CAD build for the part. Positions are in the model's coordinates, mm. Face numbers are marked on the shaded views. Round coordinates to 2 decimals unless told otherwise and drop trailing zeros. Loops run counter-clockwise (first coordinate to the right, second up) from the corner with the lowest first, then second, coordinate; pieces in that order, holes last. Notation, with made-up numbers: M 37.5,60 L 65.5,60 A12 ccw 65.5,73 Z; hole C 79.25,-5 d3. An arc over 180 degrees is marked long. One line per item, written item: value. Start each with the question number.
from build123d import *

# Parameters (mm, degrees)
ESQUISSE1_W             = 120
ESQUISSE1_H             = 120
BOSS_EXTRU_2_DEPTH      = 5
ESQUISSE9_R             = 4
BOSS_EXTRU_4_DEPTH      = 37.5
CHANFREIN5_SIZE         = 15
CHANFREIN6_SIZE         = 15
CHANFREIN7_SIZE         = 15
CHANFREIN8_SIZE         = 15
D_GAGEMENT_61_D         = 2.75
D_GAGEMENT_61_DEPTH     = 15
D_GAGEMENT_61_TIP       = 0.826183351
ESQUISSE21_W            = 90
ESQUISSE21_H            = 5
BOSS_EXTRU_7_DEPTH      = 40
ESQUISSE22_W            = 90
ESQUISSE22_H            = 5
BOSS_EXTRU_8_DEPTH      = 40
CHANFREIN23_SIZE        = 20
ESQUISSE23_R            = 2
ENL_V_MAT_EXTRU_1_DEPTH = 10
SKETCH1_W               = 10
SKETCH1_H               = 55
CUT_EXTRUDE2_DEPTH      = 5
FILLET2_R               = 5
FILLET3_R               = 5
SKETCH3_W               = 10
SKETCH3_H               = 55
CUT_EXTRUDE4_DEPTH      = 5
FILLET11_R              = 5
SKETCH2_W               = 8
SKETCH2_H               = 55
CUT_EXTRUDE5_DEPTH      = 8
SKETCH4_W               = 8
SKETCH4_H               = 55
CUT_EXTRUDE6_DEPTH      = 8
FILLET12_R              = 4
FILLET13_R              = 6
FILLET14_R              = 4
FILLET15_R              = 4
SKETCH5_W               = 3
SKETCH5_H               = 40
BOSS_EXTRUDE1_DEPTH     = 20
CHAMFER1_SIZE           = 10
CHAMFER2_SIZE           = 10


# Some blends are built 0.0001 mm under size
with BuildPart() as part:
    # Esquisse1 → Boss.-Extru.2 (new body)
    with BuildSketch(Plane.XY):
        with Locations((18.92806479, -29.794391972)):
            Rectangle(ESQUISSE1_W, ESQUISSE1_H)
    extrude(amount=BOSS_EXTRU_2_DEPTH)

    # Esquisse9 → Boss.-Extru.4 (add)
    with BuildSketch(Plane.XY.offset(5)):
        with Locations(Location((-22.57193521, -64.794391972, 0), (0, 0, 180))):
            Circle(ESQUISSE9_R)
        with Locations(Location((-22.57193521, 0.205608028, 0), (0, 0, 180))):
            Circle(ESQUISSE9_R)
        with Locations(Location((60.42806479, 0.205608028, 0), (0, 0, 180))):
            Circle(ESQUISSE9_R)
        with Locations(Location((60.42806479, -64.794391972, 0), (0, 0, 180))):
            Circle(ESQUISSE9_R)
    extrude(amount=BOSS_EXTRU_4_DEPTH)

    # Chanfrein5
    chanfrein5_edges = [part.edges().sort_by_distance(p)[0] for p in [
        (78.92806479, -89.794391972, 2.5),
    ]]
    chamfer(chanfrein5_edges, length=CHANFREIN5_SIZE)

    # Chanfrein6
    chanfrein6_edges = [part.edges().sort_by_distance(p)[0] for p in [
        (78.92806479, 30.205608028, 2.5),
    ]]
    chamfer(chanfrein6_edges, length=CHANFREIN6_SIZE)

    # Chanfrein7
    chanfrein7_edges = [part.edges().sort_by_distance(p)[0] for p in [
        (-41.07193521, 30.205608028, 2.5),
    ]]
    chamfer(chanfrein7_edges, length=CHANFREIN7_SIZE)

    # Chanfrein8
    chanfrein8_edges = [part.edges().sort_by_distance(p)[0] for p in [
        (-41.07193521, -89.794391972, 2.5),
    ]]
    chamfer(chanfrein8_edges, length=CHANFREIN8_SIZE)

    # Dégagement #61
    with Locations(Plane(origin=(-22.57193521, -64.794391972, 42.5), x_dir=(1, 0, 0), z_dir=(0, 0, 1))):
        with Locations((0, 0), (83, 0), (83, 65), (0, 65)):
            Hole(D_GAGEMENT_61_D / 2, depth=D_GAGEMENT_61_DEPTH)
            with Locations((0, 0, -(D_GAGEMENT_61_DEPTH + D_GAGEMENT_61_TIP / 2))):  # 118° drill point
                Cone(0, D_GAGEMENT_61_D / 2, D_GAGEMENT_61_TIP, mode=Mode.SUBTRACT)

    # Esquisse21 → Boss.-Extru.7 (add)
    with BuildSketch(Plane(origin=(0, -89.794391972, 0), x_dir=(-1, 0, 0), z_dir=(0, -1, 0))):
        with Locations((-18.92806479, -2.5)):
            Rectangle(ESQUISSE21_W, ESQUISSE21_H)
    extrude(amount=BOSS_EXTRU_7_DEPTH)

    # Esquisse22 → Boss.-Extru.8 (add)
    with BuildSketch(Plane(origin=(0, 30.205608028, 0), x_dir=(1, 0, 0), z_dir=(0, 1, 0))):
        with Locations((18.92806479, -2.5)):
            Rectangle(ESQUISSE22_W, ESQUISSE22_H)
    extrude(amount=BOSS_EXTRU_8_DEPTH)

    # Chanfrein23
    chanfrein23_edges = [part.edges().sort_by_distance(p)[0] for p in [
        (-26.07193521, -129.794391972, 2.5),
        (63.92806479, -129.794391972, 2.5),
        (63.92806479, 70.205608028, 2.5),
        (-26.07193521, 70.205608028, 2.5),
    ]]
    chamfer(chanfrein23_edges, length=CHANFREIN23_SIZE)

    # Esquisse23 → Enlèv. mat.-Extru.1 (cut)
    with BuildSketch(Plane.XY.offset(5)):
        with Locations((-35.996277988, -74.213194945)):
            Circle(ESQUISSE23_R)
        with Locations((-26.096783051, -84.112689881)):
            Circle(ESQUISSE23_R)
        with Locations((-25.52408096, 25.096608028)):
            Circle(ESQUISSE23_R)
        with Locations((-35.390089468, 15.163739554)):
            Circle(ESQUISSE23_R)
        with Locations((63.953155144, 24.523663425)):
            Circle(ESQUISSE23_R)
        with Locations((73.85265008, 14.624168488)):
            Circle(ESQUISSE23_R)
        with Locations((63.953210541, -84.112391972)):
            Circle(ESQUISSE23_R)
        with Locations((73.852705477, -74.212897035)):
            Circle(ESQUISSE23_R)
    extrude(amount=-ENL_V_MAT_EXTRU_1_DEPTH, mode=Mode.SUBTRACT)

    # Sketch1 → Cut-Extrude2 (cut)
    with BuildSketch(Plane.XY.offset(5)):
        with Locations((18.92806479, -80.294391972)):
            Rectangle(SKETCH1_W, SKETCH1_H)
    extrude(amount=-CUT_EXTRUDE2_DEPTH, mode=Mode.SUBTRACT)

    # Fillet2
    fillet2_edges = [part.edges().sort_by_distance(p)[0] for p in [
        (13.92806479, -107.794391972, 2.5),
    ]]
    fillet(fillet2_edges, radius=FILLET2_R)

    # Fillet3
    fillet3_edges = [part.edges().sort_by_distance(p)[0] for p in [
        (13.92806479, -52.794391972, 2.5),
        (23.92806479, -52.794391972, 2.5),
        (23.92806479, -107.794391972, 2.5),
    ]]
    fillet(fillet3_edges, radius=FILLET3_R - 0.0001)  # a hair under: the kernel refuses the full size

    # Sketch3 → Cut-Extrude4 (cut)
    with BuildSketch(Plane.XY.offset(5)):
        with Locations((18.92806479, 36.166130895)):
            Rectangle(SKETCH3_W, SKETCH3_H)
    extrude(amount=-CUT_EXTRUDE4_DEPTH, mode=Mode.SUBTRACT)

    # Fillet11
    fillet11_edges = [part.edges().sort_by_distance(p)[0] for p in [
        (13.92806479, 63.666130895, 2.5),
        (23.92806479, 63.666130895, 2.5),
        (23.92806479, 8.666130895, 2.5),
        (13.92806479, 8.666130895, 2.5),
    ]]
    fillet(fillet11_edges, radius=FILLET11_R - 0.0001)  # a hair under: the kernel refuses the full size

    # Sketch2 → Cut-Extrude5 (cut)
    with BuildSketch(Plane.XY.offset(5)):
        with Locations((37.92806479, -68.710279878)):
            Rectangle(SKETCH2_W, SKETCH2_H)
        with Locations((-0.07193521, -68.710279878)):
            Rectangle(SKETCH2_W, SKETCH2_H)
    extrude(amount=-CUT_EXTRUDE5_DEPTH, mode=Mode.SUBTRACT)

    # Sketch4 → Cut-Extrude6 (cut)
    with BuildSketch(Plane.XY.offset(5)):
        with Locations((-0.07193521, 23.705608028)):
            Rectangle(SKETCH4_W, SKETCH4_H)
        with Locations((37.92806479, 23.705608028)):
            Rectangle(SKETCH4_W, SKETCH4_H)
    extrude(amount=-CUT_EXTRUDE6_DEPTH, mode=Mode.SUBTRACT)

    # Fillet12
    fillet12_edges = [part.edges().sort_by_distance(p)[0] for p in [
        (33.92806479, 51.205608028, 2.5),
        (41.92806479, 51.205608028, 2.5),
        (41.92806479, -3.794391972, 2.5),
        (33.92806479, -3.794391972, 2.5),
    ]]
    fillet(fillet12_edges, radius=FILLET12_R - 0.0001)  # a hair under: the kernel refuses the full size

    # Fillet13
    # the kernel refuses this fillet: 6 mm, written as the material it adds along each edge
    with BuildSketch(Plane(origin=(-4.07193521, -3.794391972, 5), x_dir=(1, 0, 0), z_dir=(0, 0, -1)), Plane(origin=(3.92806479, -3.794391972, 5), x_dir=(0, 1, 0), z_dir=(0, 0, -1)), Plane(origin=(-4.07193521, 51.205608028, 5), x_dir=(0, -1, 0), z_dir=(0, 0, -1))) as fillet13_piece_1:
        with BuildLine():
            CenterArc((FILLET13_R, -FILLET13_R), FILLET13_R, 90, 90)
            Line((0, -FILLET13_R), (0, 0))
            Line((0, 0), (FILLET13_R, 0))
        make_face()
    extrude(amount=5)
    with BuildSketch(Plane(origin=(3.92806479, 51.205608028, 5), x_dir=(0, -1, 0), z_dir=(0, 0, -1))) as fillet13_piece_2:
        with BuildLine():
            CenterArc((FILLET13_R, FILLET13_R), FILLET13_R, 180, 90)
            Line((0, FILLET13_R), (0, 0))
            Line((0, 0), (FILLET13_R, 0))
        make_face()
    extrude(amount=5)

    # Fillet14
    fillet14_edges = [part.edges().sort_by_distance(p)[0] for p in [
        (3.92806479, -41.210279878, 2.5),
        (-4.07193521, -41.210279878, 2.5),
        (-4.07193521, -96.210279878, 2.5),
        (3.92806479, -96.210279878, 2.5),
    ]]
    fillet(fillet14_edges, radius=FILLET14_R - 0.0001)  # a hair under: the kernel refuses the full size

    # Fillet15
    fillet15_edges = [part.edges().sort_by_distance(p)[0] for p in [
        (41.92806479, -96.210279878, 2.5),
        (33.92806479, -96.210279878, 2.5),
        (33.92806479, -41.210279878, 2.5),
        (41.92806479, -41.210279878, 2.5),
    ]]
    fillet(fillet15_edges, radius=FILLET15_R - 0.0001)  # a hair under: the kernel refuses the full size

    # Sketch5 → Boss-Extrude1 (add)
    with BuildSketch(Plane.XY.offset(5)):
        with Locations((-9.57193521, -29.794391972)):
            Rectangle(SKETCH5_W, SKETCH5_H)
        with Locations((47.42806479, -29.794391972)):
            Rectangle(SKETCH5_W, SKETCH5_H)
    extrude(amount=BOSS_EXTRUDE1_DEPTH)

    # Chamfer1
    chamfer1_edges = [part.edges().sort_by_distance(p)[0] for p in [
        (47.42806479, -9.794391972, 25),
    ]]
    chamfer(chamfer1_edges, length=CHAMFER1_SIZE)

    # Chamfer2
    chamfer2_edges = [part.edges().sort_by_distance(p)[0] for p in [
        (-9.57193521, -9.794391972, 25),
    ]]
    chamfer(chamfer2_edges, length=CHAMFER2_SIZE)


solid = part.part
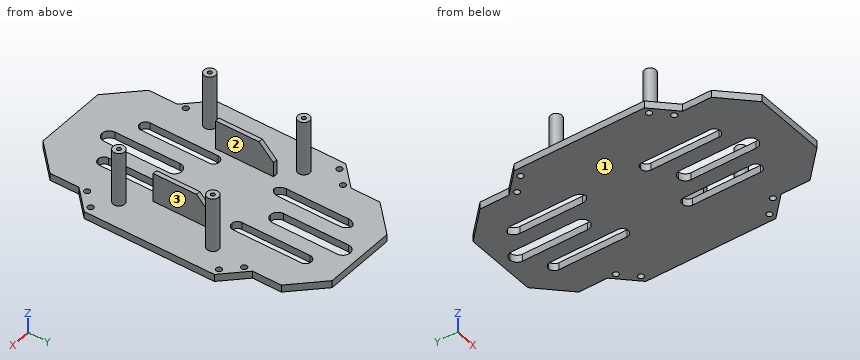
(1) Mould opens along X. For the marked faces 1, 2 and 3 say: pulls with the +X half, pulls with the -X half, needs draft (parallel to the pull), parting line crosses it, or undercut.
(2) Probe L1, parallel to X at y = -22, z = 23.5; L2, parallel to Z at x = 67, y = 24.5; L3, parallel to X at y = -68, z = 16. List the from-to ranges inside material, lowest first.
(3) Slice it at B-B, the plane z = 35. List the corners of the cut face in (x, y) (3 decimals).
(4) Slice it at C-C, the plane z = 19.5. List the corners of the cut face in (x, y), and give its area (3 significant figures).
(5) Slice it at D-D, the plane x = 6. List the corners of the cut face in (y, z), and give its area (3 significant figures).
(6) Slice it at A-A, the plane y = 42. List the corners of the cut face in (x, z).
(7) Flat gauge pins, fed straight in: P1, Ø4, axis at y = -78.5, z = 3, coming from the -X side; P2, Ø10, axis at y = -44.5, z = 13.5, coming from the -X side; P3, Ø3.5, axis at x = -9, z = 11, coming from the +Y side. Where does each tip first touch, or does it go through?
Check result:
1. face 1: needs draft
1. face 2: undercut
1. face 3: pulls with the +X half
2. L1: x = -11.07 to -8.07, 45.93 to 48.93
2. L2: z = 0 to 5
2. L3: x = -24.96 to -20.18, 58.04 to 62.82
3. outline: C -22.572,-64.794 d8; C -22.572,0.206 d8; C 60.428,-64.794 d8; C 60.428,0.206 d8; hole C -22.572,-64.794 d2.75; hole C -22.572,0.206 d2.75; hole C 60.428,-64.794 d2.75; hole C 60.428,0.206 d2.75
4. outline: C -22.57,-64.79 d8; C -22.57,0.21 d8; M -11.07,-49.79 L -8.07,-49.79 L -8.07,-14.29 L -11.07,-14.29 Z; M 45.93,-49.79 L 48.93,-49.79 L 48.93,-14.29 L 45.93,-14.29 Z; C 60.43,-64.79 d8; C 60.43,0.21 d8
4. area: 414 mm^2
5. outline: M -129.79,0 L 70.21,0 L 70.21,5 L -129.79,5 Z
5. area: 1,000 mm^2
6. outline: M -26.07,0 L -4.07,0 L -4.07,5 L -26.07,5 Z; M 3.93,0 L 13.93,0 L 13.93,5 L 3.93,5 Z; M 23.93,0 L 33.93,0 L 33.93,5 L 23.93,5 Z; M 41.93,0 L 63.93,0 L 63.93,5 L 41.93,5 Z
7. P1: stops at x = -39.37
7. P2: stops at x = -11.07
7. P3: stops at y = -9.79
